Input: dimensioned drawing with shaded views. Units: mm. Origin: part minimum x, y, z. Coordinates: 2 decimals unless noted, no trailing zeros. Write each loop counter-clockwise with the first axis right and the second up, starting at its lowest first coordinate (ties: lowest second). Pieces come first, ordered by that corner, then holes. Notation, with made-up numbers: M -38,71.25 L -17,71.25 A20 cw -17,82.25 Z; hole C -19,-14 d1. An arc over 180 degrees is marked long. Use one line per item in the form item = value.
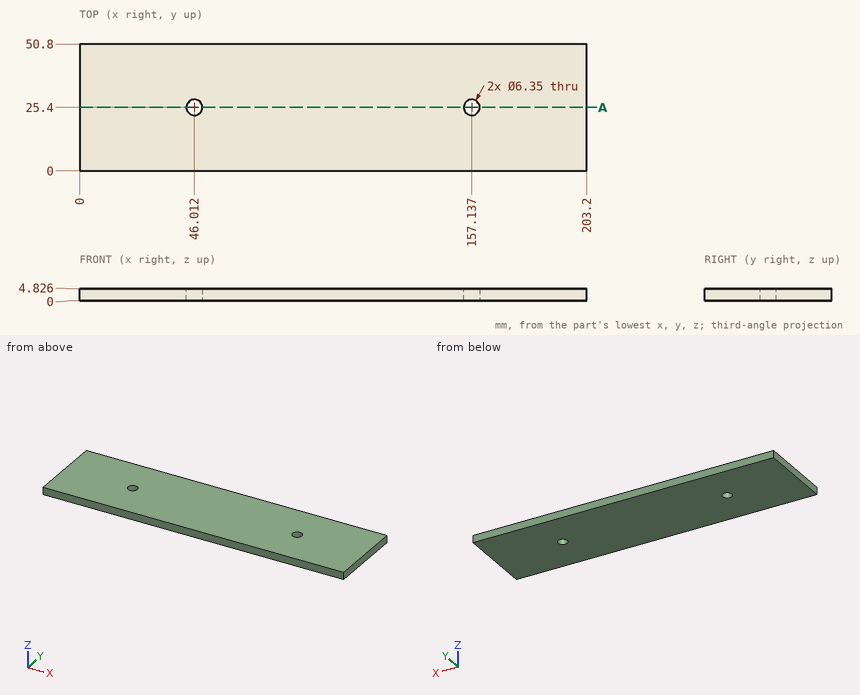
(1) First-contact query: pin 1 Ø1.5 at (y, z) = (43, 3.5) entering from -X. Flat tip, straight axial feed; report the tip coordinate or a pass-through.
Computed:
pin_1 = 0
(2) Line query: probe 1 along Y at (x, z) = (155, 0.5); probe 2 along Y at (x, z) = (43.5, 2.25). Output: solid intervals per line, ascending.
Computed:
probe_1 = 0 to 23.05, 27.75 to 50.8
probe_2 = 0 to 23.46, 27.34 to 50.8
(3) Section query A-A on y = 25.4. Return the cut outline in (x, z), plus the area to 3 significant figures.
Computed:
outline = M 0,0 L 42.84,0 L 42.84,4.83 L 0,4.83 Z; M 49.19,0 L 153.96,0 L 153.96,4.83 L 49.19,4.83 Z; M 160.31,0 L 203.2,0 L 203.2,4.83 L 160.31,4.83 Z
area = 919 mm^2
